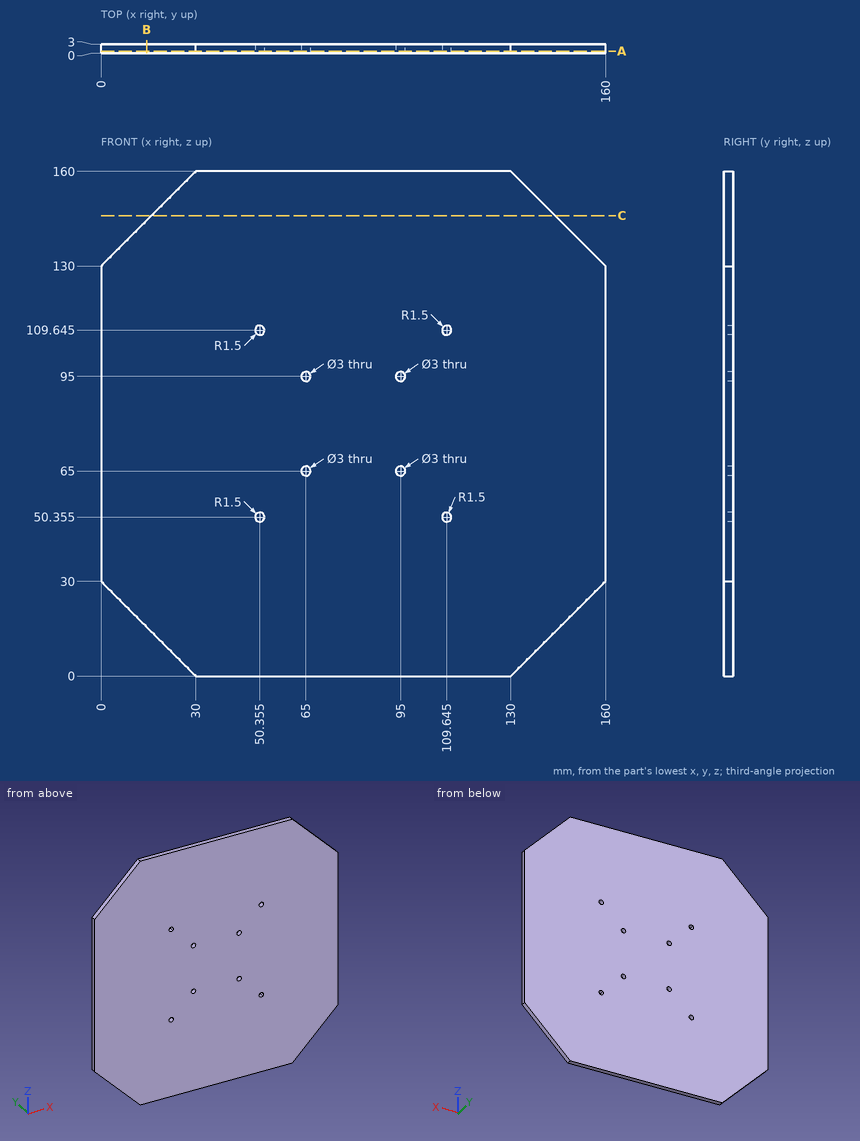
Drawing for the job (mm, zero at the part's lowest x, y, z). Coordinates: 2 decimals unless noted, no trailing zeros. Order: outer loops, then holes, each group sorted by start corner. A loop starts at its lowest first (then second) coordinate and runs counter-clockwise, first axis right, second up. Notation, with made-up numbers: (69, 55) - (100, 55) arc R21 ccw to (100, 90) - close; hole circle Ø10 at (87, 63.5). An arc over 180 degrees is marked (long way). Use a Markdown table: item, result. Add a question column.
(1) Saw through at A-A (y = 0.75). Count the separate pieces of the cut face and the enclosed holes in it, then the cut area to 3 significant figures.
(2) Flat gauge pins, fed straight in: pin 1 (1.5 mm diameter, centred on x = 59, z = 30, fed in from -Y); pin 2 (2.5 mm diameter, centred on x = 95, z = 95, fed in from -Y). Where does each tip first touch, or does it go through?
(3) Drill centre lines: line 1 along X through (y, z) = (0.8, 95); line 2 along Z through (x, y) = (110, 0.65). Where is each one in solid material? Low to high. Write a range as [from, to].
(4) Saw through at B-B (x = 14.5). Give the cut face in (y, z), then the cut area to 3 significant figures.
(5) Saw through at C-C (z = 146). Give the cut face in (x, y), then the cut area to 3 significant figures.
Solved:
| question | item | result |
|---|---|---|
| 1 | separate pieces | 1 |
| 1 | enclosed holes | 8 |
| 1 | area | 23,700 mm² |
| 2 | pin 1 | stops at y = 0 |
| 2 | pin 2 | passes through |
| 3 | line 1 | x = [0, 63.5], [66.5, 93.5], [96.5, 160] |
| 3 | line 2 | z = [0, 48.9], [51.81, 108.19], [111.1, 160] |
| 4 | outline | (0, 15.5) - (3, 15.5) - (3, 144.5) - (0, 144.5) - close |
| 4 | area | 387 mm² |
| 5 | outline | (16, 0) - (144, 0) - (144, 3) - (16, 3) - close |
| 5 | area | 384 mm² |
